from build123d import *

# Parameters (mm, degrees)
SKETCH1_R           = 1.5
BOSS_EXTRUDE1_DEPTH = 5
SKETCH2_R           = 2.940597014
BOSS_EXTRUDE2_DEPTH = 2
FILLET1_R           = 1


with BuildPart() as part:
    # Sketch1 → Boss-Extrude1 (new body)
    with BuildSketch(Plane.XY):
        Circle(SKETCH1_R)
    extrude(amount=BOSS_EXTRUDE1_DEPTH)

    # Sketch2 → Boss-Extrude2 (add)
    with BuildSketch(Plane.XY.offset(5)):
        Circle(SKETCH2_R)
    extrude(amount=BOSS_EXTRUDE2_DEPTH)

    # Fillet1
    fillet1_edges = [part.edges().sort_by_distance(p)[0] for p in [
        (-2.940597014, 0, 7),
    ]]
    fillet(fillet1_edges, radius=FILLET1_R)


solid = part.part
For this review, take the finished solid that the model builds, in its own axes (mm). A direction names the side the tool comes from. Give positions to 0.01 mm unless a question says otherwise; leave off trailing zeros. Loops run counter-clockwise (first coordinate to the right, second up) from the corner with the lowest first, then second, coordinate; pieces in that order, holes last. Notation, with made-up numbers: M 69,23.5 L 76,23.5 A15 ccw 76,43.5 Z; hole C 78,11 d2. An arc over 180 degrees is marked long. Put each result on its own line as item: value. Start each with the question number.
(1) Add section A-A, the plane y = 0. Write out the cut boundary in (x, z), then the cut area to 3 significant figures.
(2) Machinability: for faces 1 (the flat face through (0, 0, 7)), 2 (the cylindrical face through (-1.5, 0.07, 2.46)), which of the approach directions +Z, -Z, +X, -X, +Y, -Y give a long, thin tool a straight path to every point of the face, cutting with its end or side? Answer none if there is none.
(3) Add section C-C, the plane z = 5.75. Write out the cut boundary in (x, y), then the cut area to 3 significant figures.
(4) Add section D-D, the plane z = 3. Write out the cut boundary in (x, y), then the cut area to 3 significant figures.
(5) Wall thickness on L1, parallel to Z at x = 0.1, y = 1.9; L2, parallel to Y at x = 0.05, z = 3.5; L3, parallel to X at y = 2.35, z = 5.5: over which ranges is each line inside the solid? List them lowest first.
(6) For pin 1 (1.5 mm diameter, centred on y = -1, z = 4.5, fed in from +X), flat-tipped, find the tip position at first contact; note if it passes through.
Result:
1. outline: M -2.94,5 L -1.5,5 L -1.5,0 L 1.5,0 L 1.5,5 L 2.94,5 L 2.94,6 A1 ccw 1.94,7 L -1.94,7 A1 ccw -2.94,6 Z
1. area: 26.3 mm^2
2. face 1: +Z, +X, -X, +Y, -Y
2. face 2: -Z
3. outline: C 0,0 d5.88
3. area: 27.2 mm^2
4. outline: C 0,0 d3
4. area: 7.07 mm^2
5. L1: z = 5 to 7
5. L2: y = -1.5 to 1.5
5. L3: x = -1.77 to 1.77
6. pin 1: stops at x = 2.91
